from build123d import *

# Parameters (mm, degrees)
SKETCH1_W           = 1830
SKETCH1_H           = 130
BOSS_EXTRUDE1_DEPTH = 175
SKETCH4_R           = 12.75
CUT_EXTRUDE1_DEPTH  = 64
SHELL1_START        = -55
SHELL1_OUTLINE_W    = 1810
SHELL1_OUTLINE_H    = 335
SHELL1_OUTLINE_R    = 22.75
SHELL1_DEPTH        = 110
SHELL1_START_2      = 9
SHELL1_2_OUTLINE_R  = 22.75
SHELL1_2_DEPTH      = 46
SKETCH5_R           = 20
CUT_EXTRUDE2_DEPTH  = 64
SKETCH6_R           = 20
CUT_EXTRUDE4_DEPTH  = 39
SKETCH7_R           = 20
CUT_EXTRUDE5_DEPTH  = 50
SKETCH9_R           = 20
CUT_EXTRUDE6_DEPTH  = 50


with BuildPart() as part:
    # Sketch1 → Boss-Extrude1 (new, symmetric)
    with BuildSketch(Plane(origin=(0, 0, 0), x_dir=(1, 0, 0), z_dir=(0, 1, 0))):
        Rectangle(SKETCH1_W, SKETCH1_H)
    extrude(amount=BOSS_EXTRUDE1_DEPTH, both=True)

    # Sketch4 → Cut-Extrude1 (cut)
    with BuildSketch(Plane(origin=(0, 0, -65), x_dir=(-1, 0, 0), z_dir=(0, 0, -1))):
        with Locations((-699.9, 80)):
            Circle(SKETCH4_R)
        with Locations((-619.9, 80)):
            Circle(SKETCH4_R)
        with Locations((-259.9, 80)):
            Circle(SKETCH4_R)
        with Locations((-179.9, 80)):
            Circle(SKETCH4_R)
        with Locations((180.1, 80)):
            Circle(SKETCH4_R)
        with Locations((260.1, 80)):
            Circle(SKETCH4_R)
        with Locations((620.1, 80)):
            Circle(SKETCH4_R)
        with Locations((700.1, 80)):
            Circle(SKETCH4_R)
    extrude(amount=-CUT_EXTRUDE1_DEPTH, mode=Mode.SUBTRACT)

    # Shell1: read off the stored shape, not the designer's step
    # Shell1 outline → Shell1 (cut)
    with BuildSketch(Plane.XY.offset(SHELL1_START)):
        with Locations((0, 2.5)):
            Rectangle(SHELL1_OUTLINE_W, SHELL1_OUTLINE_H)
        with Locations((-700.1, 80)):
            Circle(SHELL1_OUTLINE_R, mode=Mode.SUBTRACT)
        with Locations((-620.1, 80)):
            Circle(SHELL1_OUTLINE_R, mode=Mode.SUBTRACT)
        with Locations((-260.1, 80)):
            Circle(SHELL1_OUTLINE_R, mode=Mode.SUBTRACT)
        with Locations((-180.1, 80)):
            Circle(SHELL1_OUTLINE_R, mode=Mode.SUBTRACT)
        with Locations((179.9, 80)):
            Circle(SHELL1_OUTLINE_R, mode=Mode.SUBTRACT)
        with Locations((259.9, 80)):
            Circle(SHELL1_OUTLINE_R, mode=Mode.SUBTRACT)
        with Locations((619.9, 80)):
            Circle(SHELL1_OUTLINE_R, mode=Mode.SUBTRACT)
        with Locations((699.9, 80)):
            Circle(SHELL1_OUTLINE_R, mode=Mode.SUBTRACT)
    extrude(amount=SHELL1_DEPTH, mode=Mode.SUBTRACT)

    # Shell1 2 outline → Shell1 2 (cut)
    with BuildSketch(Plane.XY.offset(SHELL1_START_2)):
        with Locations((-700.1, 80)):
            Circle(SHELL1_2_OUTLINE_R)
        with Locations((-620.1, 80)):
            Circle(SHELL1_2_OUTLINE_R)
        with Locations((-260.1, 80)):
            Circle(SHELL1_2_OUTLINE_R)
        with Locations((-180.1, 80)):
            Circle(SHELL1_2_OUTLINE_R)
        with Locations((179.9, 80)):
            Circle(SHELL1_2_OUTLINE_R)
        with Locations((259.9, 80)):
            Circle(SHELL1_2_OUTLINE_R)
        with Locations((619.9, 80)):
            Circle(SHELL1_2_OUTLINE_R)
        with Locations((699.9, 80)):
            Circle(SHELL1_2_OUTLINE_R)
    extrude(amount=SHELL1_2_DEPTH, mode=Mode.SUBTRACT)

    # Sketch5 → Cut-Extrude2 (cut)
    with BuildSketch(Plane(origin=(0, 175, 0), x_dir=(1, 0, 0), z_dir=(0, 1, 0))):
        with Locations(Location((815, 0, 0), (0, 0, 270))):
            Circle(SKETCH5_R)
    extrude(amount=-CUT_EXTRUDE2_DEPTH, mode=Mode.SUBTRACT)

    # Sketch6 → Cut-Extrude4 (cut)
    with BuildSketch(Plane.ZY.offset(915)):
        with Locations((0, -50)):
            Circle(SKETCH6_R)
    extrude(amount=-CUT_EXTRUDE4_DEPTH, mode=Mode.SUBTRACT)

    # Sketch7 → Cut-Extrude5 (cut)
    with BuildSketch(Plane(origin=(0, 175, 0), x_dir=(1, 0, 0), z_dir=(0, 1, 0))):
        with Locations(Location((662.9, 0.1, 0), (0, 0, 270))):
            Circle(SKETCH7_R)
        with Locations(Location((217.3, 0.1, 0), (0, 0, 270))):
            Circle(SKETCH7_R)
        with Locations(Location((-227.5, 0.1, 0), (0, 0, 270))):
            Circle(SKETCH7_R)
        with Locations(Location((-673.4, 0.1, 0), (0, 0, 270))):
            Circle(SKETCH7_R)
    extrude(amount=-CUT_EXTRUDE5_DEPTH, mode=Mode.SUBTRACT)

    # Sketch9 → Cut-Extrude6 (cut)
    with BuildSketch(Plane(origin=(915, 0, 0), x_dir=(0, 0, -1), z_dir=(1, 0, 0))):
        with Locations((0.1, -98.5)):
            Circle(SKETCH9_R)
    extrude(amount=-CUT_EXTRUDE6_DEPTH, mode=Mode.SUBTRACT)


solid = part.part
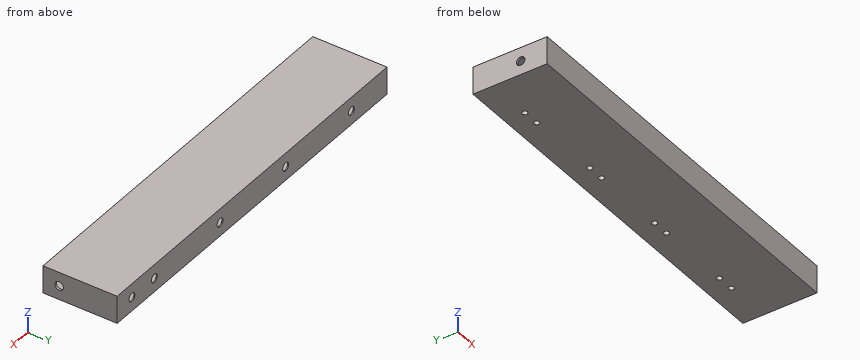
Could you check a few things on this model? Use its own coordinates, in mm. Coordinates: 2 decimals unless noted, no trailing zeros. Loops run counter-clockwise (first coordinate to the right, second up) from the corner with the lowest first, then second, coordinate; pieces in that order, holes last.
1. Imagine slicing it at A-A (z = 35). Please give me the cut outline in (x, y), and give its area (4 significant figures).
2. Imagine slicing it at B-B (x = 311). Please give me the cut outline in (y, z), and give its area (3 significant figures).
3. For P1, Ø7.5, axis at x = 178, y = 86, coming from the -Z side, with a flat end and sliding along its axis, tell me the tip position at first contact or that it passes through.
4. I need wall thicknesses on L1, parallel to Y at x = -620.1, z = -14; L2, parallel to Z at x = 257, y = 47; L3, parallel to X at y = 171, z = 0. Which ranges of each line are inside material? Lowest first, please.
5. Imagine slicing it at C-C (y = -50). Please give me the cut outline in (x, z).
Computed values:
1. outline: (-915, -175) - (915, -175) - (915, 175) - (-915, 175) - close; hole (-905, -165) - (905, -165) - (905, 170) - (-905, 170) - close
1. area: 34,150 mm2
2. outline: (-175, -65) - (175, -65) - (175, 65) - (-175, 65) - close; hole (-165, -55) - (170, -55) - (170, 55) - (-165, 55) - close
2. area: 8,650 mm2
3. P1: stops at z = -1
4. L1: y = -175 to -165, 57.25 to 67.25, 92.75 to 102.75, 170 to 175
4. L2: z = -65 to -55, 55 to 65
4. L3: x = -915 to -693.4, -653.4 to -247.5, -207.5 to 197.3, 237.3 to 642.9, 682.9 to 795, 835 to 915
5. outline: (-915, -65) - (915, -65) - (915, 65) - (-915, 65) - (-915, 20) - (-905, 20) - (-905, 55) - (905, 55) - (905, -55) - (-905, -55) - (-905, -20) - (-915, -20) - close
